from build123d import *

# Parameters (mm, degrees)
SKETCH1_W           = 6.35
SKETCH1_H           = 0.396875
BOSS_EXTRUDE1_DEPTH = 12.7


with BuildPart() as part:
    # Sketch1 → Boss-Extrude1 (new body)
    with BuildSketch(Plane(origin=(0, 0, 0), x_dir=(1, 0, 0), z_dir=(0, 1, 0))):
        Polygon((-13.335, 6.35), (-13.335, -15.875), (0, -15.875), (0, -12.7), (-10.16, -12.7), (-10.16, 6.35), align=None)
        Polygon((0, -12.7), (0, -15.875), (3.175, -15.875), (3.175, -0.396875), (3.175, 0), (0, 0), align=None)
        with Locations((6.35, -0.1984375)):
            Rectangle(SKETCH1_W, SKETCH1_H)
    extrude(amount=BOSS_EXTRUDE1_DEPTH)


solid = part.part
CAD build for the part. Positions are in the model's coordinates, mm. A direction names the side the tool comes from. Coordinates: 2 decimals unless noted, no trailing zeros. Write each loop counter-clockwise with the first axis right and the second up, starting at its lowest first coordinate (ties: lowest second). Pieces come first, ordered by that corner, then holes. Notation, with made-up numbers: (-32, 83) - (26, 83) arc R17 ccw to (26, 90) - close; hole circle Ø9 at (-19.5, 5.25). An arc over 180 degrees is marked (long way). Use a Markdown table: item, result. Add a question column.
Item 1: Band-saw the part on B-B, the plane y = 2. Give the cut face in (x, z) (3 decimals), and give its area (3 significant figures).
Item 2: 3-axis set-ups, long thin cutter, end or side, ignore diameter. For faces 1 (the face through (-5, 6, 12.7)), 2 (the face through (-10.4, 0, 8)), 3 (the face through (-12, 6, -6.35)), 4 (the face through (5, 6, 0)), 5 (the face through (3.175, 6, 8)): which of +Z, -Z, +X, -X, +Y, -Y reach the whole face in a straight line?
Item 3: Band-saw the part on C-C, the plane x = -2. Give the cut face in (y, z) (3 decimals), and give its area (3 significant figures).
Item 4: Band-saw the part on A-A, the plane z = 2.25. Give the cut face in (x, y) (3 decimals).
Item 5: Mould opens along X. For faces 6 (the face through (0, 6, 6)), 7 (the face through (-5, 6, 15.875)), 8 (the face through (-13.335, 6, 5)) say: pulls with the +X half, pulls with the -X half, needs draft (parallel to the pull), parting line crosses it, or undercut.
Item 6: Flat gauge pins, fed straight in: pin 1 (7.5 mm diameter, centred on x = 4.5, y = 7, fed in from -Z); pin 2 (4 mm diameter, centred on y = 9, z = 8, fed in from +X) (3 decimals); pin 3 (5 mm diameter, centred on x = -3, y = 6, fed in from -Z). Where does each tip first touch, or does it go through?
Item 7: Band-saw the part on D-D, the plane z = -0.75. Give the cut face in (x, y) (3 decimals), and give its area (3 significant figures).
Item 8: Drill centre lines: L1, parallel to X at y = 0.5, z = 3.25 (3 decimals); L2, parallel to X at y = 6.5, z = 13.75 (3 decimals); L3, parallel to Z at x = 5.5, y = 8.5. Where is each one in solid material? Low to high. Write a range as from..to.
Numbers:
| question | item | result |
|---|---|---|
| 1 | outline | (-13.335, -6.35) - (-10.16, -6.35) - (-10.16, 12.7) - (0, 12.7) - (0, 0) - (9.525, 0) - (9.525, 0.397) - (3.175, 0.397) - (3.175, 15.875) - (-13.335, 15.875) - close |
| 1 | area | 156 mm2 |
| 2 | face 1 | -Z, +Y, -Y |
| 2 | face 2 | +Z, -Z, +X, -X, -Y |
| 2 | face 3 | -Z, +X, -X, +Y, -Y |
| 2 | face 4 | -Z, +X, +Y, -Y |
| 2 | face 5 | +Z, +X, +Y, -Y |
| 3 | outline | (0, 12.7) - (12.7, 12.7) - (12.7, 15.875) - (0, 15.875) - close |
| 3 | area | 40.3 mm2 |
| 4 | outline | (-13.335, 0) - (-10.16, 0) - (-10.16, 12.7) - (-13.335, 12.7) - close; (0, 0) - (3.175, 0) - (3.175, 12.7) - (0, 12.7) - close |
| 5 | face 6 | undercut |
| 5 | face 7 | needs draft |
| 5 | face 8 | pulls with the -X half |
| 6 | pin 1 | z = 0 |
| 6 | pin 2 | x = 3.175 |
| 6 | pin 3 | z = 12.7 |
| 7 | outline | (-13.335, 0) - (-10.16, 0) - (-10.16, 12.7) - (-13.335, 12.7) - close |
| 7 | area | 40.3 mm2 |
| 8 | L1 | -13.335..-10.16, 0..3.175 |
| 8 | L2 | -13.335..3.175 |
| 8 | L3 | 0..0.4 |
